Autodesk Inventor part; units mm, degrees
ref_plane "YZ Plane" through (0, 0, 0) normal (1, 0, 0) x (0, 1, 0)
ref_plane "XZ Plane" through (0, 0, 0) normal (0, 1, 0) x (-1, 0, 0)
ref_plane "XY Plane" through (0, 0, 0) normal (0, 0, 1) x (1, 0, 0)
sketch "Sketch1" plane through (0, 0, 0) normal (0, 1, 0) x (-1, 0, 0)
  line L0 (0, 0) -> (16, 0)
  line L1 (16, 0) -> (16, -91)
  line L2 (16, -91) -> (0, -91)
  line L3 (0, -91) -> (0, 0)
  dimension "d0" = 16
  dimension "d1" = 91
extrude "Extrusion1" add sketch "Sketch1" along normal blind 25
sketch "Sketch2" plane through (0, 25, 0) normal (0, 1, 0) x (1, 0, 0)
  line L0 (-16, 91) -> (-16, 0)
  circle A0 centre (-16, 12.8045) radius 4
  circle A1 centre (-16, 57.8045) radius 4
  point P0 (0, 0)
  dimension "d4" = 8
  dimension "d5" = 8
  dimension "d6" = 45
extrude "Extrusion2" cut sketch "Sketch2" against normal blind 20
sketch "Sketch3" plane through (0, 25, 0) normal (0, 1, 0) x (1, 0, 0)
  circle A0 centre (-7, 6.5) radius 2
  circle A1 centre (-7, 84.5) radius 2
  line L0 (-16, 8.8045) -> (-16, 0)
  line L1 (-16, 53.8045) -> (-16, 16.8045)
  line L2 (-16, 8.8045) -> (-16, 61.8045)
  point P0 (0, 0)
  point P1 (-16, 3)
  point P2 (-16, 88)
  dimension "d10" = 4
  dimension "d12" = 4
  dimension "d15" = 9
  dimension "d17" = 9
  dimension "d18" = 6.5
ref_plane "Work Plane1" through (0, 0, -3) normal (1, 0, 0) x (0, 0, -1)
sketch "Sketch4" plane through (0, 0, -3) normal (1, 0, 0) x (0, 0, -1)
  circle A0 centre (17.9995, 19.5) radius 2
  circle A1 centre (69.9995, 19.5) radius 2
  line L0 (-3, 0) -> (88, 0)
  dimension "d21" = 4
  dimension "d22" = 4
  dimension "d34" = 52
  dimension "d59" = 19.5
  dimension "d60" = 19.5
extrude "Extrusion4" cut sketch "Sketch4" against normal blind 30
sketch "Sketch5" plane through (-16, 0, -91) normal (-1, 0, 0) x (0, 0, 1)
  point P0 (91, 0)
sketch "Sketch6" plane through (-16, 0, -91) normal (-1, 0, 0) x (0, 0, 1)
  arc A0 (46.1955, 15) -> (65.1955, 15) centre (55.6955, 15) ccw
  line L0 (37.1955, 25) -> (37.1955, 5)
  line L1 (37.1955, 25) -> (74.1955, 25)
  line L2 (46.1955, 15) -> (46.1955, 30.0529)
  line L3 (46.1955, 30.0529) -> (65.1955, 30.0529)
  line L4 (65.1955, 30.0529) -> (65.1955, 15)
  point P0 (91, 0)
  dimension "d25" = 19
  dimension "d26" = 18.5
  dimension "d27" = 10
extrude "Extrusion5" cut sketch "Sketch6" against normal blind 8.5
sketch "Sketch7" plane through (-7.5, 0, -91) normal (-1, 0, 0) x (0, 0, 1)
  circle A0 centre (55.6955, 15) radius 2.75
  line L0 (37.1955, 25) -> (37.1955, 5)
  point P0 (91, 0)
  dimension "d30" = 5.5
  dimension "d31" = 18.5
extrude "Extrusion6" cut sketch "Sketch7" against normal blind 30
sketch "Sketch9" plane through (0, 25, 0) normal (0, 1, 0) x (1, 0, 0)
  line L0 (0, 14.304) -> (-3.5, 14.304)
  line L1 (-3.5, 14.304) -> (-3.5, 56.304)
  line L2 (-3.5, 56.304) -> (0, 56.304)
  line L3 (0, 56.304) -> (0, 14.304)
  line L4 (-16, 0) -> (0, 0)
  dimension "d48" = 3.5
  dimension "d49" = 42
  dimension "d50" = 14.304
extrude "Extrusion7" add sketch "Sketch9" along normal blind 10
sketch "Sketch8" plane through (0, 0, 0) normal (1, 0, 0) x (0, 0, -1)
  circle A0 centre (19.8045, -0.5) radius 1.8
  circle A1 centre (50.8045, -0.5) radius 1.8
  circle A2 centre (50.8045, 30.5) radius 1.8
  circle A3 centre (19.8045, 30.5) radius 1.8
  circle A4 centre (35.3045, 15) radius 2.75
  circle A5 centre (35.3045, 15) radius 11.5
  point P0 (0, 0)
  dimension "d35" = 3.6
  dimension "d36" = 3.6
  dimension "d37" = 3.6
  dimension "d38" = 3.6
  dimension "d39" = 31
  dimension "d40" = 31
  dimension "d41" = 31
  dimension "d42" = 31
  dimension "d43" = 0
  dimension "d44" = 23
  dimension "d45" = 15.5
  dimension "d46" = 15.5
  dimension "d47" = 0
extrude "Extrusion8" cut sketch "Sketch8" against normal blind 10 contours A0 | A1 | A2 | A3
extrude "Extrusion9" cut sketch "Sketch8" against normal blind 3 contours A5
extrude "Extrusion10" cut sketch "Sketch3" against normal blind 30
properties part number "motorradrod"
Could you check a few things on this model? Use its own coordinates, in mm. A direction names the side the tool comes from. Give positions to 0.01 mm unless a question says otherwise; leave off trailing zeros. Order: outer loops, then holes, each group sorted by start corner. A loop starts at its lowest first (then second) coordinate and runs counter-clockwise, first axis right, second up.
1. Suppose I cut it at B-B (x = -6.5). List the corners of the cut face in (y, z) for me.
2. We'd pull the mould along Y, two halves only. Please class faces 1 (the cylindrical face through (-1.726, 32.285, -19.57)), 2 (the flat face through (-16, 12, -45)), 3 (the flat face through (-14, 5, -58)): pulls with the +Y half, pulls with the -Y half, needs draft (parallel to the pull), parting line crosses it, or undercut.
3. Suppose I cut it at A-A (y = 19.5). List the corners of the cut face in (x, z) for me, plus the area to 3 significant figures.
4. Suppose I cut it at D-D (x = -13). List the corners of the cut face in (y, z) for me.
5. Will these pins go through, and if not, where does the flat tip stop? P1, Ø1, axis at x = -5, z = -18.5, coming from the +Y side; P2, Ø2.5, axis at y = 19.5, z = -21, coming from the +X side; P3, Ø8, axis at y = 28.5, z = -42.5, coming from the -X side; P4, Ø4, axis at x = -2.5, y = 32, coming from the +Z side.
6. I need wall thicknesses on L1, parallel to Z at x = -7, y = 7.75; L2, parallel to Z at x = -7, y = 13; L3, parallel to Z at x = -5.75, y = 8. Which ranges of each line are inside material? Lowest first, please.
7. For faces 4 (the flat face through (-3.5, 30, -35)), 5 (the cylindrical face through (-11.81, 5.502, -35.513)), 6 (the cylindrical face through (-4.9, 1.3, -50.8)), 7 (the flat face through (-2, 30, -14.304)), 8 (the flat face through (-2, 30, -56.304)), which set-ups out of +Z, -Z, +X, -X, +Y, -Y let a thin tool reach every point of the face, with its end or its side?
8. Suppose I cut it at C-C (z = -51). List the corners of the cut face in (x, y) for me.
Solved:
1. outline: (0, -91) - (25, -91) - (25, -86.44) - (0, -86.44) - close; (0, -82.56) - (25, -82.56) - (25, -8.44) - (0, -8.44) - (0, -18.08) arc R1.8 cw to (0, -21.53) - (0, -49.08) arc R1.8 cw to (0, -52.53) - close; (0, -4.56) - (25, -4.56) - (25, 0) - (0, 0) - close; hole circle Ø5.5 at (15, -35.3); hole circle Ø4 at (19.5, -73); hole circle Ø4 at (19.5, -21)
2. face 1: undercut
2. face 2: needs draft
2. face 3: pulls with the +Y half
3. outline: (-16, -91) - (0, -91) - (0, -75) - (-16, -75) - close; (-16, -71) - (0, -71) - (0, -45.89) - (-3, -45.89) - (-3, -24.72) - (0, -24.72) - (0, -23) - (-16, -23) - (-16, -25.8) - (-7.5, -25.8) - (-7.5, -44.8) - (-16, -44.8) - (-16, -53.8) arc R4 cw to (-16, -61.8) - close; (-16, -19) - (0, -19) - (0, 0) - (-16, 0) - (-16, -8.8) arc R4 cw to (-16, -16.8) - close; hole circle Ø4 at (-7, -84.5); hole circle Ø4 at (-7, -6.5)
3. area: 1,030 mm2
4. outline: (0, -91) - (25, -91) - (25, -60.45) - (5, -60.45) - (5, -55.16) - (25, -55.16) - (25, -44.8) - (15, -44.8) arc R9.5 cw to (15, -25.8) - (25, -25.8) - (25, -15.45) - (5, -15.45) - (5, -10.16) - (25, -10.16) - (25, 0) - (0, 0) - close; hole circle Ø4 at (19.5, -73); hole circle Ø4 at (19.5, -21)
5. P1: stops at y = 25
5. P2: passes through
5. P3: stops at x = -7.5
5. P4: stops at z = -14.3
6. L1: z = -91 to -86.5, -82.5 to -8.5, -4.5 to 0
6. L2: z = -91 to -86.5, -82.5 to -37.19, -33.42 to -8.5, -4.5 to 0
6. L3: z = -91 to -86.06, -82.94 to -8.06, -4.94 to 0
7. face 4: +Z, -Z, -X, +Y
7. face 5: -X, +Y
7. face 6: +X, -Y
7. face 7: +Z, +X, -X, +Y
7. face 8: -Z, +X, -X, +Y
8. outline: (-16, 0) - (-10, 0) - (-10, 1.29) - (0, 1.29) - (0, 28.71) - (-3.5, 28.71) - (-3.5, 25) - (-16, 25) - close; (-3.5, 32.29) - (0, 32.29) - (0, 35) - (-3.5, 35) - close
